Source: CAD feature listing. Evaluate the final solid. Frame: model axes, mm. A direction names the side the tool comes from. Give positions to 0.01 mm unless a question says otherwise; leave off trailing zeros. Write each loop counter-clockwise with the first axis right and the second up, starting at its lowest first coordinate (ties: lowest second). Pieces come first, ordered by that corner, then holes. Notation, with made-up numbers: M 45.5,52.5 L 98.5,52.5 A11 cw 98.5,68.5 Z; hole C 21.5,0 d6. An arc over 180 degrees is marked long. Answer as a JSON object with one key per item and string values. Group by question number.
Autodesk Inventor part; units mm, degrees
ref_plane "YZ Plane" through (0, 0, 0) normal (1, 0, 0) x (0, 1, 0)
ref_plane "XZ Plane" through (0, 0, 0) normal (0, 1, 0) x (-1, 0, 0)
ref_plane "XY Plane" through (0, 0, 0) normal (0, 0, 1) x (1, 0, 0)
sketch "Boceto1" plane through (0, 0, 0) normal (0, 0, 1) x (1, 0, 0)
  line L0 (0, 0) -> (0, -127)
  line L1 (0, -130) -> (0, -127)
  line L2 (-101.4948, -130) -> (-101.4948, -133)
  line L3 (-101.4948, 3) -> (-101.4948, 0)
  line L4 (-104.4221, 0) -> (-104.4221, -130)
  line L5 (-104.4221, -133) -> (-101.4948, -133)
  line L6 (-104.4221, 3) -> (-101.4948, 3)
  line L7 (-9.639, -118) -> (-94.7832, -118)
  line L8 (-94.7832, -118) -> (-94.7832, -12)
  line L9 (-94.7832, -12) -> (-9.639, -12)
  line L10 (-9.639, -12) -> (-9.639, -118)
  line L11 (-9.639, -118) -> (-94.7832, -12) construction
  line L12 (-94.7832, -118) -> (-9.639, -12) construction
  line L13 (-104.4221, -133) -> (-104.4221, -130)
  line L14 (-104.4221, 0) -> (-104.4221, 3)
  line L15 (-101.4948, -130) -> (-101.4948, -129.7)
  line L16 (-101.4948, -129.7) -> (0, -129.7)
  line L17 (-101.4948, 0) -> (-101.4948, -0.3)
  line L18 (-101.4948, -0.3) -> (0, -0.3)
  point P0 (-2.2595, 0)
  dimension "d3" = 9.639
  dimension "d4" = 0.3
  dimension "d5" = 0.3
extrude "Extrusión1" add sketch "Boceto1" along normal blind 3
(1) Section D-D, the plane x = -8. Return loops of the section in (y, z).
(2) Section C-C, the plane y = -26. Return loops of the section in (x, z), plus the area to 3 significant figures.
(3) Section A-A, the plane x = -46. Return loops of the section in (y, z).
(4) Section B-B, the plane z = 2.2. Return loops of the section in (x, y).
(5) Pull-direction query (X, two-part tool) for faces 1 (the flat face through (-53, -12, 1)), 2 (the flat face through (-9.639, -64, 1)), 3 (the flat face through (0, -66, 1)), 4 (the flat face through (-103, -133, 1)); classes: pulls with the +X half, pulls with the -X half, needs draft (parallel to the pull), parting line crosses it, or undercut.
(6) Contact query for flat-ended pins moving along their axis: pin 1 Ø0.9 at (x, z) = (-46.5, 2) entering from -Y; pin 2 Ø0.9 at (y, z) = (1.5, 1.5) entering from +X; pin 3 Ø1 at (x, z) = (-79, 2) entering from +Y. Output: stop coordinate, or through.
(7) Access query for faces 5 (the flat face through (-51, -0.3, 1)), 6 (the flat face through (-52, -118, 1)), 7 (the flat face through (-103, 3, 1)), 8 (the flat face through (-101.495, -131, 1)). Directions: +Z, -Z, +X, -X, +Y, -Y. A direction counts if a zero-diameter tool reaches every point of the face in a straight line with its end or side. Return the directions, or none.
(8) Ray query, L1, parallel to Y at x = -39.5, z = 2.55; L2, parallel to X at y = -49.5, z = 1.85; L3, parallel to Y at x = -8, z = 0.4. Return the intervals inside material, ascending. Write a range as [from, to].
Reported:
{
 "1": {"outline": "M -129.7,0 L -0.3,0 L -0.3,3 L -129.7,3 Z"},
 "2": {"outline": "M -104.42,0 L -94.78,0 L -94.78,3 L -104.42,3 Z; M -9.64,0 L 0,0 L 0,3 L -9.64,3 Z", "area": "57.8 mm2"},
 "3": {"outline": "M -129.7,0 L -118,0 L -118,3 L -129.7,3 Z; M -12,0 L -0.3,0 L -0.3,3 L -12,3 Z"},
 "4": {"outline": "M -104.42,-133 L -101.49,-133 L -101.49,-129.7 L 0,-129.7 L 0,-0.3 L -101.49,-0.3 L -101.49,3 L -104.42,3 Z; hole M -94.78,-118 L -9.64,-118 L -9.64,-12 L -94.78,-12 Z"},
 "5": {"face 1": "undercut", "face 2": "undercut", "face 3": "pulls with the +X half", "face 4": "needs draft"},
 "6": {"pin 1": "stops at y = -129.7", "pin 2": "stops at x = -101.49", "pin 3": "stops at y = -0.3"},
 "7": {"face 5": "+Z, -Z, +X, +Y", "face 6": "+Z, -Z", "face 7": "+Z, -Z, +X, -X, +Y", "face 8": "+Z, -Z, +X, -Y"},
 "8": {"L1": "y = [-129.7, -118], [-12, -0.3]", "L2": "x = [-104.42, -94.78], [-9.64, 0]", "L3": "y = [-129.7, -0.3]"}
}
